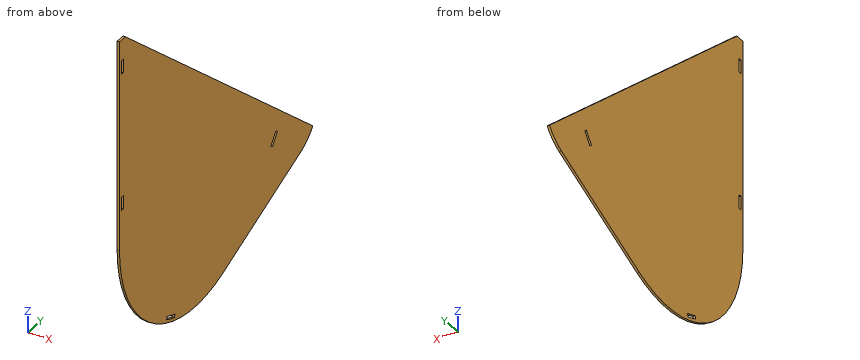
```python
from build123d import *

# Parameters (mm, degrees)
BASE_FLANGE1_DEPTH = 6
SKETCH3_W          = 35
SKETCH3_H          = 8
CUT_EXTRUDE2_DEPTH = 6


# Sheet-metal steps are written as plain solids
with BuildPart() as part:
    # Sketch1 → Base-Flange1 (new body)
    with BuildSketch(Plane(origin=(0, 0, 0), x_dir=(0, 0, -1), z_dir=(1, 0, 0))):
        with BuildLine():
            Line((691.263386145, 750.024971585), (828.145509118, 420.991908823))
            ThreePointArc((828.145509118, 420.991908823), (799.356039458, 125.196469257), (537.308857372, -15))
            Line((537.308857372, -15), (0, -15))
            Line((0, -15), (0, 10))
            Line((0, 10), (651.687076161, 800.513923243))
            ThreePointArc((651.687076161, 800.513923243), (674.911649445, 777.963121002), (691.263386145, 750.024971585))
        make_face()
    extrude(amount=-BASE_FLANGE1_DEPTH)

    # Sketch3 → Cut-Extrude2 (cut)
    with BuildSketch(Plane(origin=(0, 0, 0), x_dir=(0, 0, -1), z_dir=(1, 0, 0))):
        with BuildLine():
            Line((832.717916058, 216.438716825), (825.035135409, 218.669161062))
            ThreePointArc((825.035135409, 218.669161062), (819.970515176, 202.5140849), (813.999628283, 186.671566993))
            Line((813.999628283, 186.671566993), (821.42397234, 183.691782549))
            ThreePointArc((821.42397234, 183.691782549), (827.533179903, 199.905831283), (832.717916058, 216.438716825))
        make_face()
        with Locations((70.170932866, -3)):
            Rectangle(SKETCH3_W, SKETCH3_H)
        with Locations((421.025597194, -3)):
            Rectangle(SKETCH3_W, SKETCH3_H)
        Polygon((581.55788083, 644.957729578), (609.163726943, 623.44221749), (614.081558277, 629.752125173), (586.475712165, 651.267637261), align=None)
    extrude(amount=-CUT_EXTRUDE2_DEPTH, mode=Mode.SUBTRACT)


solid = part.part
```
Check sheet for the modelled part. Datum: model origin and axes. Units: mm. Coordinates: 2 decimals unless noted, no trailing zeros. Loops run counter-clockwise (first coordinate to the right, second up) from the corner with the lowest first, then second, coordinate; pieces in that order, holes last. Notation, with made-up numbers: M -25,44 L -13,44 A18 ccw -13,76 Z; hole C 53.5,49 d4. An arc over 180 degrees is marked long. Answer as a JSON object with one key per item and string values.
1. Scan lines: L1, parallel to Z at x = -4.95, y = 202.5; L2, parallel to Z at x = -5.25, y = 644; L3, parallel to Y at x = -5.7, z = -597. Record each from-to range of solid material in increasing order. Write a range as from..to.
Outcome:
{"L1": "-836.84..-828.41, -819.97..-158.69", "L2": "-735.37..-595.8, -582.79..-522.66", "L3": "-9.29..632.92, 643.07..734.18"}
2. Sectioned sample at B-B on y = 664. Record the cut outline in (x, z), and give its area (3 significant figures).
Outcome:
{"outline": "M -6,-727.05 L 0,-727.05 L 0,-539.15 L -6,-539.15 Z", "area": "1,130 mm²"}
3. Depth check by flat-ended pin: P1, Ø3, axis at x = -4, y = 284, coming from the -Z side; P2, Ø2, axis at x = -1, y = 444, coming from the -Z side. Enter the tip coordinate at first touch or a pass-through.
Outcome:
{"P1": "z = -851.97", "P2": "z = -818.99"}
4. Sectioned sample at C-C on z = -350.5. Record the cut outline in (x, y).
Outcome:
{"outline": "M -6,-15 L 0,-15 L 0,435.17 L -6,435.17 Z"}
5. Sectioned sample at A-A on x = -1.55. Record the cut outline in (y, z).
Outcome:
{"outline": "M -15,-537.31 A315 ccw 420.99,-828.15 L 750.02,-691.26 A120 ccw 800.51,-651.69 L 10,0 L -15,0 Z; hole M -7,-438.53 L 1,-438.53 L 1,-403.53 L -7,-403.53 Z; hole M -7,-87.67 L 1,-87.67 L 1,-52.67 L -7,-52.67 Z; hole M 183.69,-821.42 A307 ccw 216.44,-832.72 L 218.67,-825.04 A299 cw 186.67,-814 Z; hole M 623.44,-609.16 L 629.75,-614.08 L 651.27,-586.48 L 644.96,-581.56 Z"}
